Check sheet for the modelled part. Datum: model origin and axes. Units: mm. A direction names the side the tool comes from. Coordinates: 2 decimals unless noted, no trailing zeros.
from build123d import *

# Parameters (mm, degrees)
F0_W      = 800
F0_H      = 1700
F1_DEPTH  = 600
F2_T      = -40
F3_W      = 720
F3_H      = 30
F4_DEPTH  = 560
F5_R      = 39.99999
F7_DEPTH  = 560
F8_W      = 720
F8_H      = 30
F9_DEPTH  = 560
F10_W     = 720
F10_H     = 30
F11_DEPTH = 560


# Not quite as in the source:
# - a fillet or chamfer is up to 0.001 mm smaller than in the source, because OpenCascade refuses the exact size


with BuildPart() as f1:
    # F0 (on Front) → F1 (new body)
    with BuildSketch(Plane.XZ):
        Rectangle(F0_W, F0_H)
    extrude(amount=F1_DEPTH)

    # F2
    f2_openings = [f1.faces().sort_by_distance(p)[0] for p in [
        (0, -600, 0),
    ]]
    offset(amount=F2_T, openings=f2_openings)

    # F3 (on face) → F4 (join)
    with BuildSketch(Plane.XZ.offset(40)):
        with Locations((0, -255)):
            Rectangle(F3_W, F3_H)
    extrude(amount=F4_DEPTH)

    # F5 (radius 40 in the source; OpenCascade refuses exactly that, so slightly less here)
    f5_edges = [f1.edges().sort_by_distance(p)[0] for p in [
        (-400, -600, 0),
        (-400, -300, 850),
        (0, -600, 850),
        (400, -300, 850),
        (0, 0, 850),
        (-400, 0, 0),
        (400, 0, 0),
        (0, 0, -850),
        (-400, -300, -850),
        (400, -300, -850),
        (0, -600, -850),
        (400, -600, 0),
    ]]
    fillet(f5_edges, radius=F5_R)

    # F6 (on face) → F7 (join)
    with BuildSketch(Plane.XZ.offset(40)):
        Polygon((360, 40), (-360, 40), (-360, 20.5096974969), (-360, 10), (360, 10), align=None)
    extrude(amount=F7_DEPTH)

    # F8 (on face) → F9 (join)
    with BuildSketch(Plane.XZ.offset(40)):
        with Locations((0, -535)):
            Rectangle(F8_W, F8_H)
    extrude(amount=F9_DEPTH)

    # F10 (on face) → F11 (join)
    with BuildSketch(Plane.XZ.offset(40)):
        with Locations((0, 305)):
            Rectangle(F10_W, F10_H)
        with Locations((0, 555)):
            Rectangle(F10_W, F10_H)
    extrude(amount=F11_DEPTH)


solid = f1.part
(1) Cross-section at A-A (y = -389). Count the separate pieces of the cut face and the enclosed holes in it, and give its area (3 significant figures).
Filled in:
separate pieces: 1
enclosed holes: 6
area: 300,000 mm2
(2) Tool access check on faces 5 (the flat face through (360, -316, 688)), 6 (the flat face through (-2, -600, 304)). Record the directions out of +Z, -Z, +X, -X, +Y, -Y that give a thin tool (end or side, any length) a straight path to the whole face; none if there is none.
Filled in:
face 5: -Y
face 6: +Z, -Z, +X, -X, -Y
(3) Thickness scan on probe 1 along X at (y, z) = (-498, 84.5); probe 2 along X at (y, z) = (-565, 421.5); probe 3 along Y at (x, z) = (292.5, 461.5). Record the ranges inside material, lowest first.
Filled in:
probe 1: x = -400 to -360, 360 to 400
probe 2: x = -399.69 to -360, 360 to 399.69
probe 3: y = -40 to 0
(4) Go/stop test with a flat-tipped pin: P1, Ø1.5, axis at x = -79.5, z = 183.5, coming from the -Y side. Record where the tip stops, or that it passes through.
Filled in:
P1: stops at y = -40
(5) Release check for a two-part mould opening along Z. For faces 1 (the flat face through (-360, -316, 163)), 2 (the cylindrical face through (387.972, -303.64, -838.594)), 3 (the flat face through (-5, -296, 850)), 4 (the flat face through (-5, -316, 540)) record: +Z half, -Z half, draft (parallel to the pull), parting line (faces both ways), or undercut.
Filled in:
face 1: undercut
face 2: -Z half
face 3: +Z half
face 4: undercut
